Could you check a few things on this drawing? It's one solid part, dimensions in mm from its lowest x, y, z. A direction names the side the tool comes from. Coordinates: 2 decimals unless noted, no trailing zeros. Write each loop counter-clockwise with the first axis right and the second up, starting at its lowest first coordinate (ties: lowest second). Pieces come first, ordered by that corner, then holes. Notation, with made-up numbers: (29.5, 19) - (73.5, 19) arc R34 cw to (73.5, 55) - close; hole circle Ø2 at (38.5, -29). An arc over 180 degrees is marked (long way). Use one line per item in the form item = value. Start each with the question number.
(1) Thinking about a two-plate mould opening in Y: for the marked faces 1, 2 and 3, which applies, pulls with the +Y half, pulls with the -Y half, needs draft (parallel to the pull), parting line crosses it, or undercut?
(2) On a 3-axis mill with a long thin cutter (end or side, diameter ignored), from which of +Z, -Z, +X, -X, +Y, -Y can I reach the whole of each face in a straight line? I mean the marked faces 4 and 5. Say none if no direction works.
(3) If we section it at C-C on y = 36: Please give me the cut outline in (x, z).
(4) If we section it at A-A on x = 25: Please give me the cut outline in (y, z), then the cut area to 3 significant figures.
(5) If we section it at D-D on z = 4.75: Give the number of separate pieces and of enclosed holes in the cut face, then the cut area to 3 significant figures.
(6) If we section it at B-B on x = 34: Please give me the cut outline in (y, z).
(7) For pin 1 Ø3.5 at (x, z) = (10, 4) entering from +Y; pin 2 Ø5 at (x, y) = (25, 44.5) entering from +Z, each with a flat end and sliding along its axis, tell me the tip position at first contact or that it passes through.
(8) If I drill on probe 1 along Y at (x, z) = (25, 5.6); probe 2 along X at (y, z) = (10, 3); probe 3 along Y at (x, z) = (7.5, 6.7), over which ranges is the centre line in solid material (lowest first)? Write a range as from..to.
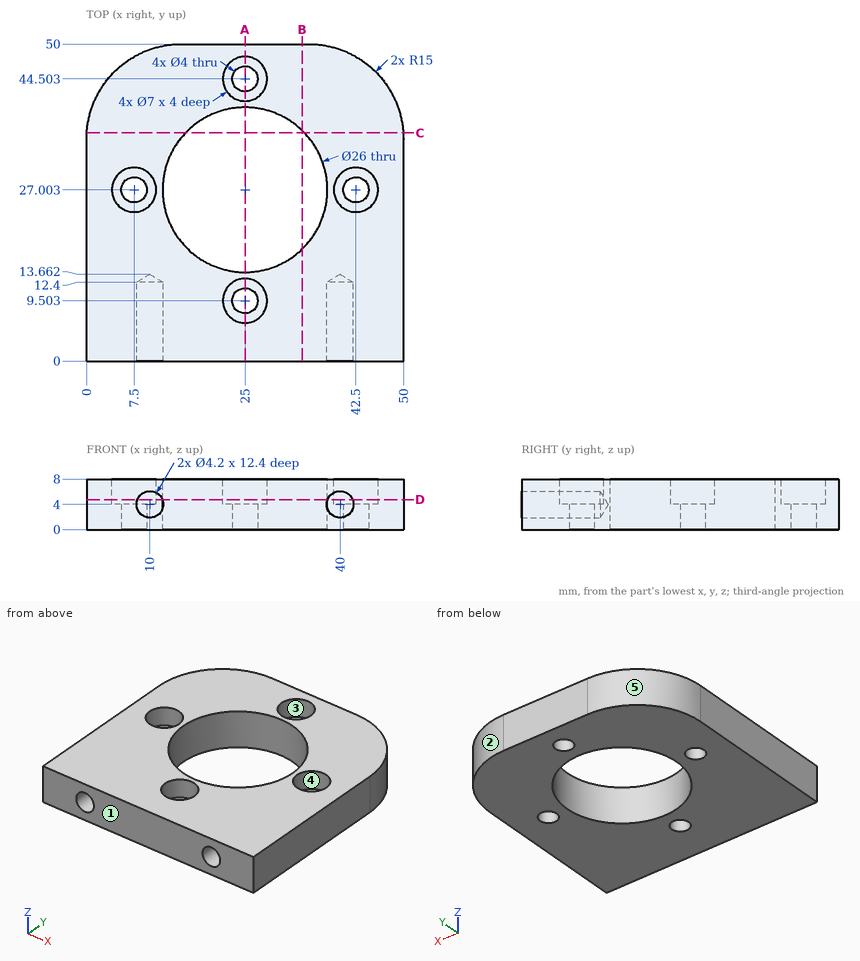
Reported:
q1.face_1 = pulls with the -Y half
q1.face_2 = pulls with the +Y half
q1.face_3 = undercut
q2.face_4 = +Z
q2.face_5 = +Z, -Z, -X, +Y
q3.outline = (0.03, 0) - (15.62, 0) - (15.62, 8) - (0.03, 8) - close; (34.38, 0) - (49.97, 0) - (49.97, 8) - (34.38, 8) - close
q4.outline = (0, 0) - (7.5, 0) - (7.5, 4) - (6, 4) - (6, 8) - (0, 8) - close; (11.5, 0) - (14, 0) - (14, 8) - (13, 8) - (13, 4) - (11.5, 4) - close; (40, 0) - (42.5, 0) - (42.5, 4) - (41, 4) - (41, 8) - (40, 8) - close; (46.5, 0) - (50, 0) - (50, 8) - (48, 8) - (48, 4) - (46.5, 4) - close
q4.area = 104 mm2
q5.separate_pieces = 1
q5.enclosed_holes = 5
q5.area = 1,620 mm2
q6.outline = (0, 0) - (17.62, 0) - (17.62, 8) - (0, 8) - close; (36.38, 0) - (50, 0) - (50, 8) - (36.38, 8) - close
q7.pin_1 = 49.64
q7.pin_2 = 4
q8.probe_1 = 0..6, 13..14, 40..41, 48..50
q8.probe_2 = 0..8.15, 11.85..23.06, 26.94..38.15, 41.85..50
q8.probe_3 = 0..23.5, 30.5..47.99
